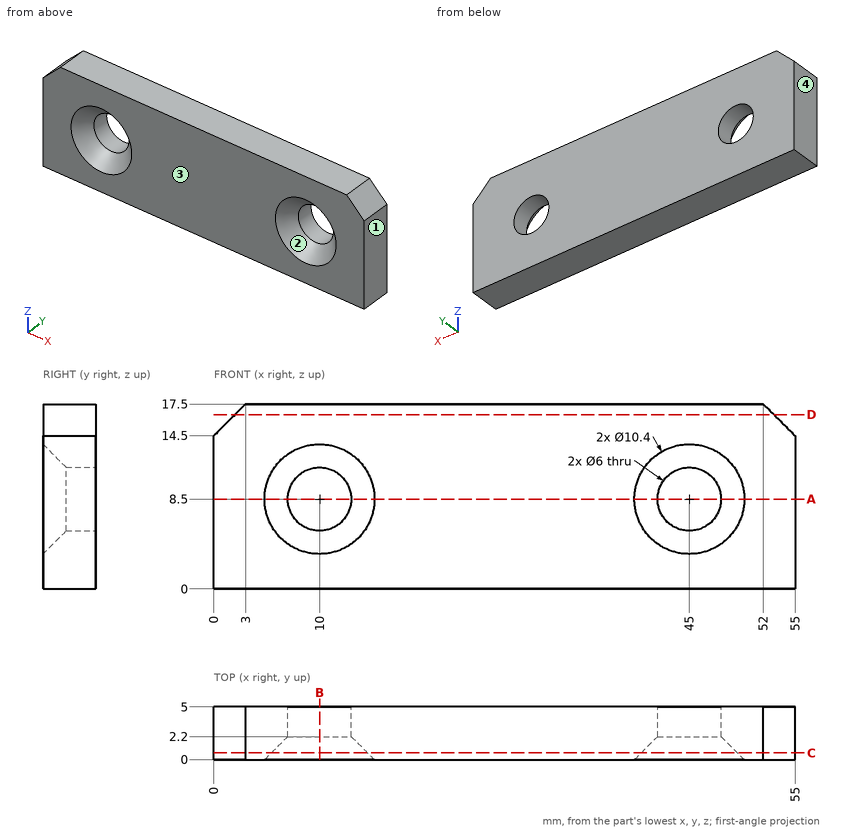
Geometry: see drawing. Coordinates: mm, zero at the bounding-box minimum. Round coordinates to 2 decimals unless told otherwise and drop trailing zeros. Loops run counter-clockwise (first coordinate to the right, second up) from the corner with the lowest first, then second, coordinate; pieces in that order, holes last. Notation, with made-up numbers: M -16,19.25 L 39,19.25 A19 ccw 39,55.25 Z; hole C -34,76 d9. An arc over 180 degrees is marked long. Use a Markdown table: item, result. Add a question column.
1. Section query D-D on z = 16.5. Return the cut outline in (x, y).
2. Section query B-B on x = 10. Return the cut outline in (y, z), then the cut area to 3 significant figures.
3. Mould query, pull axis X, two halves, no side actions, for the marked faces 1, 2, 3 and 4. Classes: pulls with the +X half, pulls with the -X half, needs draft (parallel to the pull), parting line crosses it, or undercut.
4. Section query C-C on y = 0.65. Return the cut outline in (x, z), then the cut area to 3 significant figures.
5. Contact query for flat-ended pins moving along their axis: P1, Ø9.5, axis at x = 45, z = 8.5, coming from the +Y side; P2, Ø9.5, axis at x = 10, z = 8.5, coming from the -Y side; P3, Ø1.5, axis at y = 4, z = 15.5, coming from the +X side. Output: stop coordinate, or through.
6. Line query: line 1 (X direction, y = 4.45, z = 8.5); line 2 (Z direction, x = 45, y = 3.5); line 3 (X direction, y = 3.4, z = 6.5). Output: solid intervals per line, ascending.
7. Section query A-A on z = 8.5. Return the cut outline in (x, y), then the cut area to 3 significant figures.
Reported:
| question | item | result |
|---|---|---|
| 1 | outline | M 2,0 L 53,0 L 53,5 L 2,5 Z |
| 2 | outline | M 0,0 L 5,0 L 5,5.5 L 2.2,5.5 L 0,3.3 Z; M 0,13.7 L 2.2,11.5 L 5,11.5 L 5,17.5 L 0,17.5 Z |
| 2 | area | 52.7 mm² |
| 3 | face 1 | pulls with the +X half |
| 3 | face 2 | undercut |
| 3 | face 3 | needs draft |
| 3 | face 4 | pulls with the -X half |
| 4 | outline | M 0,0 L 55,0 L 55,14.5 L 52,17.5 L 3,17.5 L 0,14.5 Z; hole C 10,8.5 d9.1; hole C 45,8.5 d9.1 |
| 4 | area | 823 mm² |
| 5 | P1 | stops at y = 5 |
| 5 | P2 | stops at y = 0.45 |
| 5 | P3 | stops at x = 54.75 |
| 6 | line 1 | x = 0 to 7, 13 to 42, 48 to 55 |
| 6 | line 2 | z = 0 to 5.5, 11.5 to 17.5 |
| 6 | line 3 | x = 0 to 7.76, 12.24 to 42.76, 47.24 to 55 |
| 7 | outline | M 0,0 L 4.8,0 L 7,2.2 L 7,5 L 0,5 Z; M 13,2.2 L 15.2,0 L 39.8,0 L 42,2.2 L 42,5 L 13,5 Z; M 48,2.2 L 50.2,0 L 55,0 L 55,5 L 48,5 Z |
| 7 | area | 205 mm² |
